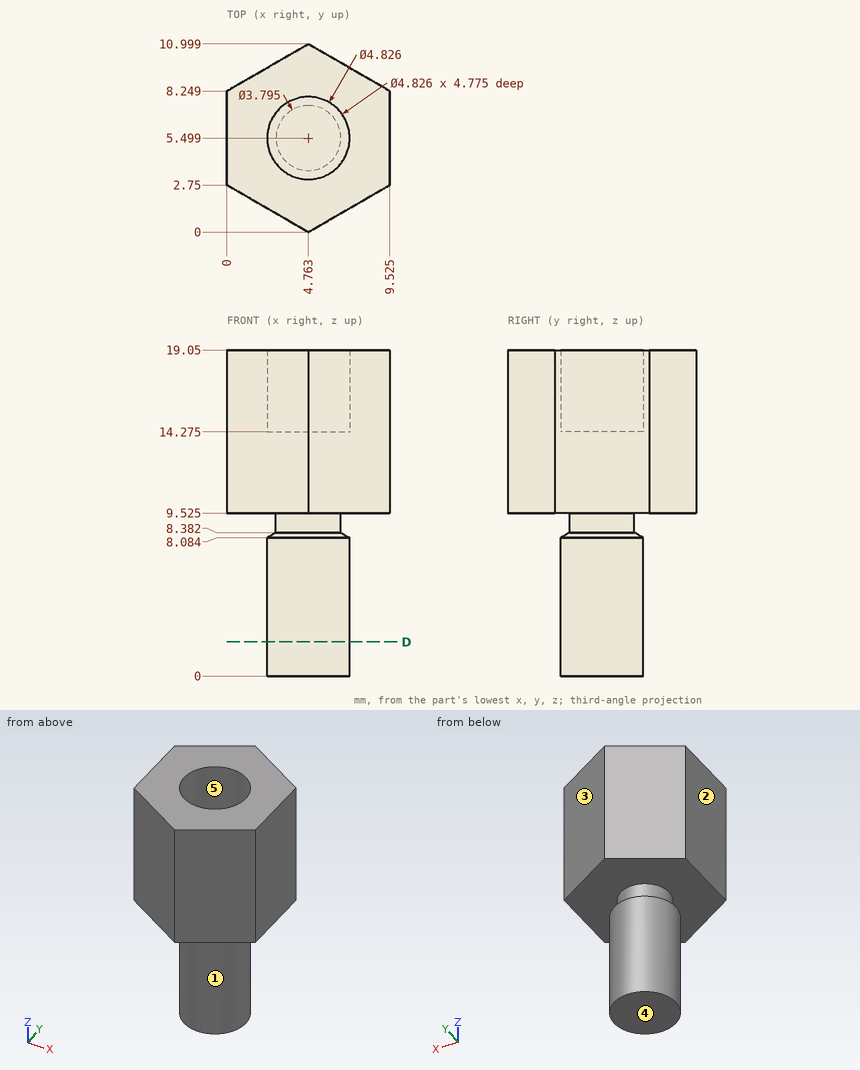
Answer from the drawing. Dimensions are ordinates in mm from the lowest x, y and z of the part. A direction names the side the tool comes from. Give positions to 0.01 mm unless a question says otherwise; leave off trailing zeros. Order: outer loops, then holes, each group sorted by start corner. A loop starts at its lowest first (then second) coordinate and runs counter-clockwise, first axis right, second up.
Item 1: Which of the six approach directions +Z, -Z, +X, -X, +Y, -Y give full straight-line access (tool end or side, diameter ignored) to the marked faces 1 and 2?
From the geometry:
face 1: -Z
face 2: +Z, -Z, -X, +Y, -Y
Item 2: Given pin 1 Ø4 at (x, y) = (4.76, 5.5) entering from +Z (1 decimal); pin 2 Ø3 at (x, y) = (5.5, 6.5) entering from -Z; pin 3 Ø2 at (y, z) = (8, 4) entering from -X, each flat-ended and moving along its own axis, determine where each tip first touches the part or whether it passes through.
From the geometry:
pin 1: stops at z = 14.3
pin 2: stops at z = 0
pin 3: stops at x = 2.87
Item 3: For a pull along X with two mould halves and no side action, classify the marked faces 3, 4 and 5 as pulls with the +X half, pulls with the -X half, needs draft (parallel to the pull), parting line crosses it, or undercut.
From the geometry:
face 3: pulls with the +X half
face 4: needs draft
face 5: undercut
Item 4: Find the intervals of material crossed by probe 1 along Y at (x, z) = (5.5, 18.25) (1 decimal); probe 2 along X at (y, z) = (5, 14.75) (1 decimal); probe 3 along Y at (x, z) = (5.75, 15.5), in increasing order.
From the geometry:
probe 1: y = 0.4 to 3.2, 7.8 to 10.6
probe 2: x = 0 to 2.4, 7.1 to 9.5
probe 3: y = 0.57 to 3.3, 7.7 to 10.43
Item 5: The part is cut by section D-D, the plane z = 2. Give the vertices of the cut face in (x, y) (1 decimal).
From the geometry:
outline: circle Ø4.8 at (4.8, 5.5)
